Could you check a few things on this model? Use its own coordinates, in mm. Round coordinates to 2 decimals unless told otherwise and drop trailing zeros. Write each loop counter-clockwise with the first axis right and the second up, starting at its lowest first coordinate (ties: lowest second). Pieces come first, ordered by that corner, then holes. Notation, with made-up numbers: (79.25, -13.75) -> (115.25, -13.75) arc R14 cw to (115.25, -4.75) -> close; hole circle Ø10 at (45, 70). An arc over 180 degrees is marked (long way). Answer in a Markdown table with one row per item.
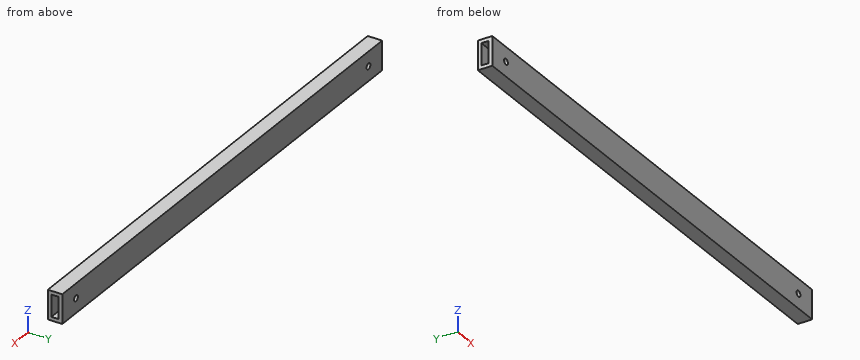
from build123d import *

# Parameters (mm, degrees)
SKETCH1_W           = 25.4
SKETCH1_H           = 12.7
SKETCH1_W_2         = 19.05
SKETCH1_H_2         = 6.35
BOSS_EXTRUDE1_DEPTH = 444.5
SKETCH2_R           = 2.667
CUT_EXTRUDE1_DEPTH  = 13.7


with BuildPart() as part:
    # Sketch1 → Boss-Extrude1 (new body)
    with BuildSketch(Plane(origin=(0, 0, 0), x_dir=(0, 0, -1), z_dir=(1, 0, 0))):
        with Locations((12.7, 6.35)):
            Rectangle(SKETCH1_W, SKETCH1_H)
        with Locations((12.7, 6.35)):
            Rectangle(SKETCH1_W_2, SKETCH1_H_2, mode=Mode.SUBTRACT)
    extrude(amount=BOSS_EXTRUDE1_DEPTH)

    # Sketch2 → Cut-Extrude1 (cut, through all)
    with BuildSketch(Plane(origin=(0, 12.7, 0), x_dir=(1, 0, 0), z_dir=(0, 1, 0))):
        with Locations((19.05, 12.7)):
            Circle(SKETCH2_R)
        with Locations((425.45, 12.7)):
            Circle(SKETCH2_R)
    extrude(amount=-CUT_EXTRUDE1_DEPTH, mode=Mode.SUBTRACT)


solid = part.part
1) Imagine slicing it at A-A, the plane y = 6. Please give me the cut outline in (x, z) (3 decimals).
Findings:
| item | result |
|---|---|
| outline | (0, -25.4) -> (444.5, -25.4) -> (444.5, -22.225) -> (0, -22.225) -> close; (0, -3.175) -> (444.5, -3.175) -> (444.5, 0) -> (0, 0) -> close |
2) For pin 1 (7 mm diameter, centred on x = 19.05, z = -12.7, fed in from -Y); pin 2 (5 mm diameter, centred on x = 425.45, z = -12.7, fed in from +Y), each with a flat end and sliding along its axis, tell me the tip position at first contact or that it passes through.
Findings:
| item | result |
|---|---|
| pin 1 | stops at y = 0 |
| pin 2 | passes through |
3) Please list where these lines run through material, in increasing order: line 1 (X direction, y = 1.15, z = -12.7); line 2 (Y direction, x = 294.5, z = -8.5) (3 decimals); line 3 (Z direction, x = 425.45, y = 10.25).
Findings:
| item | result |
|---|---|
| line 1 | x = 0 to 16.38, 21.72 to 422.78, 428.12 to 444.5 |
| line 2 | y = 0 to 3.175, 9.525 to 12.7 |
| line 3 | z = -25.4 to -15.37, -10.03 to 0 |
4) Imagine slicing it at B-B, the plane x = 283. Please give me the cut outline in (y, z) (3 decimals), plus the area to 3 significant figures.
Findings:
| item | result |
|---|---|
| outline | (0, -25.4) -> (12.7, -25.4) -> (12.7, 0) -> (0, 0) -> close; hole (3.175, -22.225) -> (9.525, -22.225) -> (9.525, -3.175) -> (3.175, -3.175) -> close |
| area | 202 mm^2 |
